Build history of the part. All positions in model axes, mm. Face numbers are marked on the shaded views. A direction names the side the tool comes from. Give positions to 0.01 mm unless a question says otherwise; leave off trailing zeros. Order: outer loops, then holes, each group sorted by start corner. A loop starts at its lowest first (then second) coordinate and runs counter-clockwise, first axis right, second up. Notation, with made-up numbers: (72.5, 23) - (118.5, 23) arc R21 cw to (118.5, 33) - close; hole circle Ø3 at (51.5, 69). An arc over 180 degrees is marked (long way). One line per item, written item: value.
```python
from build123d import *

# Parameters (mm, degrees)
F0_W      = 40
F0_H      = 33
F1_DEPTH  = 12
F2_R      = 12.65
F3_DEPTH  = 69
F4_W      = 28
F4_H      = 48.7952879344
F5_DEPTH  = 10
F7_DEPTH  = 9
F8_R      = 2.99999
F9_R      = 1.5
F10_DEPTH = 20


# Not quite as in the source:
# - a fillet or chamfer is up to 0.001 mm smaller than in the source, because OpenCascade refuses the exact size


with BuildPart() as f1:
    # F0 (on Top) → F1 (new body)
    with BuildSketch(Plane.XY):
        with Locations((-8.7267248217, -1.6879990697)):
            Rectangle(F0_W, F0_H)
    extrude(amount=F1_DEPTH)

    # F2 (on face) → F3 (cut)
    with BuildSketch(Plane.YZ.offset(11.2732751783)):
        with Locations((-1.6879990697, 14.65)):
            Circle(F2_R)
    extrude(amount=-F3_DEPTH, mode=Mode.SUBTRACT)

    # F4 (on face) → F5 (cut)
    with BuildSketch(Plane.XY.offset(12)):
        with Locations((-8.7267248217, 5.2832299843)):
            Rectangle(F4_W, F4_H)
    extrude(amount=-F5_DEPTH, mode=Mode.SUBTRACT)

    # F6 (on face) → F7 (cut)
    with BuildSketch(Plane.XY.offset(12)):
        with BuildLine():
            ThreePointArc((-25.7267248217, 9.6813178072), (-27.140938384, 9.0955313695), (-27.7267248217, 7.6813178072))
            Line((-27.7267248217, 7.6813178072), (-27.7267248217, -11.0573159465))
            ThreePointArc((-27.7267248217, -11.0573159465), (-27.140938384, -12.4715295089), (-25.7267248217, -13.0573159465))
            ThreePointArc((-25.7267248217, -13.0573159465), (-24.3125112593, -12.4715295089), (-23.7267248217, -11.0573159465))
            Line((-23.7267248217, -11.0573159465), (-23.7267248217, 7.6813178072))
            ThreePointArc((-23.7267248217, 7.6813178072), (-24.3125112593, 9.0955313695), (-25.7267248217, 9.6813178072))
        make_face()
        with BuildLine():
            ThreePointArc((8.2732751783, 9.6813178072), (6.859061616, 9.0955313695), (6.2732751783, 7.6813178072))
            Line((6.2732751783, 7.6813178072), (6.2732751783, -11.0573159465))
            ThreePointArc((6.2732751783, -11.0573159465), (6.859061616, -12.4715295089), (8.2732751783, -13.0573159465))
            ThreePointArc((8.2732751783, -13.0573159465), (9.6874887407, -12.4715295089), (10.2732751783, -11.0573159465))
            Line((10.2732751783, -11.0573159465), (10.2732751783, 7.6813178072))
            ThreePointArc((10.2732751783, 7.6813178072), (9.6874887407, 9.0955313695), (8.2732751783, 9.6813178072))
        make_face()
    extrude(amount=-F7_DEPTH, mode=Mode.SUBTRACT)

    # F8 (radius 3 in the source; OpenCascade refuses exactly that, so slightly less here)
    f8_edges = [f1.edges().sort_by_distance(p)[0] for p in [
        (5.273275, 14.812001, 7),
        (11.273275, 14.812001, 6),
        (-22.726725, 14.812001, 7),
        (-28.726725, 14.812001, 6),
        (-28.726725, -18.187999, 6),
        (-22.726725, -18.187999, 7),
        (5.273275, -18.187999, 7),
        (11.273275, -18.187999, 6),
    ]]
    fillet(f8_edges, radius=F8_R)

    # F9 (on face) → F10 (cut)
    with BuildSketch(Plane.XY.offset(12)):
        with Locations((-25.7267248217, 12.5120009303)):
            Circle(F9_R)
        with Locations((8.4634907544, 12.5120009303)):
            Circle(F9_R)
        with Locations((8.2223585095, -15.8879990697)):
            Circle(F9_R)
        with Locations((-25.7357346928, -15.8880167171)):
            Circle(F9_R)
    extrude(amount=-F10_DEPTH, mode=Mode.SUBTRACT)


solid = f1.part
```
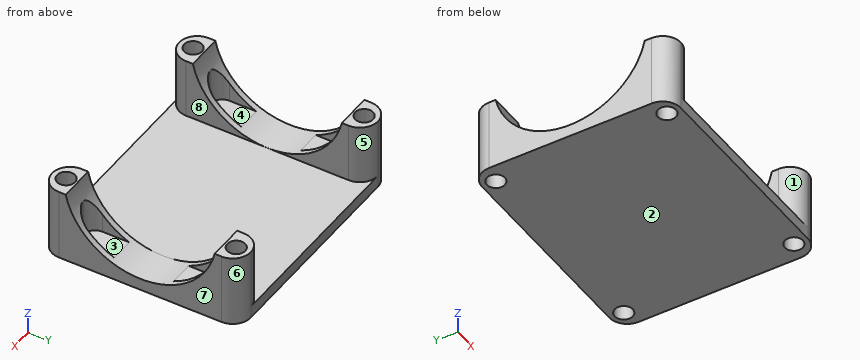
(1) Slice it at B-B, the plane y = 13.5. Give the cut face in (x, z), and give its area (3 significant figures).
Completed:
outline: (-28.21, 0) - (-26.86, 0) - (-26.86, 12) - (-28.21, 12) - close; (-24.6, 0) - (7.33, 0) - (7.33, 12) - (5.79, 12) - (5.79, 2) - (-23.25, 2) - (-23.25, 12) - (-24.6, 12) - close; (9.59, 0) - (10.75, 0) - (10.75, 12) - (9.59, 12) - close
area: 123 mm²
(2) Pin check, flat tips, straight feed: P1, Ø2, axis at x = 7.5, y = 8, coming from the +Z side; P2, Ø6, axis at y = -7.5, z = 6.5, coming from the -X side; P3, Ø5, axis at x = 2.5, z = 6, coming from the -Y side; P4, Ø3, axis at x = -5.5, y = -11, coming from the +Z side. Stop position of each tip, or through.
Completed:
P1: z = 3
P2: x = -28.73
P3: through
P4: z = 2
(3) Drill centre lines: line 1 (X direction, y = 11.5, z = 5); line 2 (Y direction, x = -26, z = 6.25); line 3 (Z direction, x = -14.5, y = -3). Where is each one in solid material? Low to high.
Completed:
line 1: -28.73 to -26.83, -24.62 to -22.73, 5.27 to 7.36, 9.57 to 11.27
line 2: -18.18 to -17.36, -14.41 to -13.04, 9.66 to 11.04, 13.99 to 14.8
line 3: 0 to 2
(4) Slice it at D-D, the plane y = -10. Give the cut face in (x, z), and give its area (3 significant figures).
Completed:
outline: (-28.73, 0) - (11.27, 0) - (11.27, 5.11) - (10.27, 5.11) - (10.27, 3) - (6.27, 3) - (6.27, 5.11) - (5.27, 5.11) - (5.27, 2) - (-22.73, 2) - (-22.73, 5.11) - (-23.73, 5.11) - (-23.73, 3) - (-27.73, 3) - (-27.73, 5.11) - (-28.73, 5.11) - close
area: 100 mm²
(5) Pull direction Y, two halves, no side cores. Call the marked faces 1, 2 and 3: +Y half, -Y half, draft (parallel to the pull), parting line (faces both ways), or undercut.
Completed:
face 1: -Y half
face 2: draft
face 3: undercut
(6) 3-axis set-ups, long thin cutter, end or side, ignore diameter. For the marked faces 4, 5, 6, 7 and 8: which of +Z, -Z, +X, -X, +Y, -Y reach the whole face in a straight line?
Completed:
face 4: +Z
face 5: +Z, +Y
face 6: +Z, -Z, +X, +Y
face 7: +Z, -Z, +X, +Y, -Y
face 8: +Z, +Y, -Y
(7) Slice it at A-A, the plane z = 2.5. Count the separate pieces of the cut face and the enclosed holes in it, and give its area (3 significant figures).
Completed:
separate pieces: 4
enclosed holes: 4
area: 268 mm²
